```python
from build123d import *

# Parameters (mm, degrees)
F0_W     = 215
F0_H     = 150
F0_R     = 1.63195
F0_R_2   = 3.96875
F0_W_2   = 124
F0_H_2   = 79
F0_R_3   = 9.525
F1_DEPTH = 1.5875
F2_R     = 4


with BuildPart() as f1:
    # F0 (on Top) → F1 (new body)
    with BuildSketch(Plane.XY):
        Rectangle(F0_W, F0_H)
        with Locations((-76.2, -66.294)):
            Circle(F0_R, mode=Mode.SUBTRACT)
        with Locations((-98.552, -38.1)):
            Circle(F0_R, mode=Mode.SUBTRACT)
        with Locations((0, -66.294)):
            Circle(F0_R, mode=Mode.SUBTRACT)
        with Locations((76.2, -66.294)):
            Circle(F0_R, mode=Mode.SUBTRACT)
        with Locations((98.552, -38.1)):
            Circle(F0_R, mode=Mode.SUBTRACT)
        with Locations((75.542, -35.53125)):
            Circle(F0_R_2, mode=Mode.SUBTRACT)
        with Locations((-20.677, 0)):
            Rectangle(F0_W_2, F0_H_2, mode=Mode.SUBTRACT)
        with Locations((-98.552, 38.1)):
            Circle(F0_R, mode=Mode.SUBTRACT)
        with Locations((-76.2, 66.294)):
            Circle(F0_R, mode=Mode.SUBTRACT)
        with Locations((65.232, 17.24805)):
            Circle(F0_R, mode=Mode.SUBTRACT)
        with Locations((85.852, 17.24805)):
            Circle(F0_R, mode=Mode.SUBTRACT)
        with Locations((75.542, 27.55805)):
            Circle(F0_R_3, mode=Mode.SUBTRACT)
        with Locations((0, 66.294)):
            Circle(F0_R, mode=Mode.SUBTRACT)
        with Locations((65.232, 37.86805)):
            Circle(F0_R, mode=Mode.SUBTRACT)
        with Locations((85.852, 37.86805)):
            Circle(F0_R, mode=Mode.SUBTRACT)
        with Locations((98.552, 38.1)):
            Circle(F0_R, mode=Mode.SUBTRACT)
        with Locations((76.2, 66.294)):
            Circle(F0_R, mode=Mode.SUBTRACT)
    extrude(amount=F1_DEPTH)

    # F2
    f2_edges = [f1.edges().sort_by_distance(p)[0] for p in [
        (-107.5, 75, 0.79375),
        (-107.5, -75, 0.79375),
        (107.5, -75, 0.79375),
        (107.5, 75, 0.79375),
    ]]
    fillet(f2_edges, radius=F2_R)


solid = f1.part
```
For this review, take the finished solid that the model builds, in its own axes (mm). Round coordinates to 2 decimals unless told otherwise and drop trailing zeros. Write each loop counter-clockwise with the first axis right and the second up, starting at its lowest first coordinate (ties: lowest second). Pieces come first, ordered by that corner, then holes. Notation, with made-up numbers: M 4,61.25 L 34,61.25 A35 ccw 34,93.25 Z; hole C 13,89 d3. An arc over 180 degrees is marked long. One line per item, written item: value. Start each with the question number.
(1) We need section A-A (x = 29). Give the boundary of the cut face in (y, z).
(2) We need section C-C (z = 0.75). Count the separate pieces of the cut face and the enclosed holes in it, and give its area (3 significant figures).
(3) We need section B-B (y = 1.5). Give the boundary of the cut face in (x, z).
(4) Wall thickness on line 1 (Y direction, x = -76.2, z = 0.75); line 2 (X direction, y = 17.5, z = 0.8); line 3 (Y direction, x = 2.5, z = 1.35): over which ranges is each line inside the solid? List them lowest first.
(5) The part is to be moulded in two halves that separate along Y. For faces 1 (the cylindrical face through (-106.359, -73.797, 0.805)), 2 (the cylindrical face through (74.682, -39.406, 0.783)), 3 (the cylindrical face through (106.297, 73.859, 0.805)), say which applies: released by +Y, released by -Y, zero draft, split by the parting line, or undercut.
Result:
1. outline: M -75,0 L -39.5,0 L -39.5,1.59 L -75,1.59 Z; M 39.5,0 L 75,0 L 75,1.59 L 39.5,1.59 Z
2. separate pieces: 1
2. enclosed holes: 17
2. area: 22,000 mm²
3. outline: M -107.5,0 L -82.68,0 L -82.68,1.59 L -107.5,1.59 Z; M 41.32,0 L 107.5,0 L 107.5,1.59 L 41.32,1.59 Z
4. line 1: -75 to -67.93, -64.66 to -39.5, 39.5 to 64.66, 67.93 to 75
4. line 2: -107.5 to -82.68, 41.32 to 63.62, 66.84 to 84.24, 87.46 to 107.5
4. line 3: -75 to -39.5, 39.5 to 75
5. face 1: released by -Y
5. face 2: undercut
5. face 3: released by +Y
